```python
from build123d import *

# Parameters (mm, degrees)
BOSS_EXTRU_2_START = 2.33
ESQUISSE3_R        = 1
BOSS_EXTRU_2_DEPTH = 2.33
ESQUISSE4_R        = 0.9
BOSS_EXTRU_3_DEPTH = 2
ESQUISSE5_W        = 0.6
ESQUISSE5_H        = 4
PER_AGE1_D         = 1.47
PER_AGE1_DEPTH     = 1.6
CHANFREIN1_SIZE    = 0.1
CONG_1_R           = 0.2


# Read off the part's stored shape, not the designer's step: Boss.-Extru.1
with BuildPart() as part:
    # Esquisse1 → Révolution1 (revolve)
    with BuildSketch(Plane(origin=(0, 0, 0), x_dir=(1, 0, 0), z_dir=(0, 1, 0))):
        Polygon((1.175, 0.5), (0, 0.5), (0, -4.02), (0.799038106, -4.02), (1, -3.27), (1, -1.054421399), (1.02, -0.979780383), (1.02, -0.946167323), (1, -0.946167323), (1, 0), (1.175, 0), align=None)
    revolve(axis=Axis((0, 0, -0.5), (0, 0, 1)))

    # Boss.-Extru.1 outline → Boss.-Extru.1 (revolve)
    with BuildSketch(Plane.XZ):
        with BuildLine():
            Line((0.6, 4.02), (0.6, 6.37))
            ThreePointArc((0.6, 6.37), (0.424264069, 6.794264069), (0, 6.97))
            Line((0, 6.97), (0, 4.02))
            Line((0, 4.02), (0.6, 4.02))
        make_face()
    revolve(axis=Axis((0, 0, 0), (0, 0, 1)))

    # Esquisse3 → Boss.-Extru.2 (add)
    with BuildSketch(Plane(origin=(0, 0, -0.5), x_dir=(-1, 0, 0), z_dir=(0, 0, -1)).offset(BOSS_EXTRU_2_START)):
        with Locations(Location((0, 0, 0), (0, 0, 180))):
            Circle(ESQUISSE3_R)
    extrude(amount=-BOSS_EXTRU_2_DEPTH)

    # Esquisse4 → Boss.-Extru.3 (add)
    with BuildSketch(Plane(origin=(0, 0, -2.83), x_dir=(-1, 0, 0), z_dir=(0, 0, -1))):
        Circle(ESQUISSE4_R)
    extrude(amount=BOSS_EXTRU_3_DEPTH)

    # Esquisse5 → Enlèvement de matière-Révolution1 (revolve, cut)
    with BuildSketch(Plane(origin=(0, 0, 0), x_dir=(1, 0, 0), z_dir=(0, 1, 0)), mode=Mode.PRIVATE) as enl_vement_de_mati_re_r_volution1_sk:
        with Locations((0.3, -1.02)):
            Rectangle(ESQUISSE5_W, ESQUISSE5_H)
    revolve(enl_vement_de_mati_re_r_volution1_sk.sketch.rotate(Axis((0, 0, -0.98), (0, 0, 1)), 90), axis=Axis((0, 0, -0.98), (0, 0, 1)), mode=Mode.SUBTRACT)

    # Perçage1
    with Locations(Plane(origin=(0, 0, -4.83), x_dir=(-1, 0, 0), z_dir=(0, 0, -1))):
        with Locations((0, 0)):
            Hole(PER_AGE1_D / 2, depth=PER_AGE1_DEPTH)

    # Chanfrein1
    chanfrein1_edges = [part.edges().sort_by_distance(p)[0] for p in [
        (-0.735, 0, -4.83),
    ]]
    chamfer(chanfrein1_edges, length=CHANFREIN1_SIZE)

    # Congé1
    cong_1_edges = [part.edges().sort_by_distance(p)[0] for p in [
        (-0.799038106, 0, 4.02),
    ]]
    fillet(cong_1_edges, radius=CONG_1_R)


solid = part.part
```
Check sheet for the modelled part. Datum: model origin and axes. Units: mm. A direction names the side the tool comes from. Round coordinates to 2 decimals unless told otherwise and drop trailing zeros. Loops run counter-clockwise (first coordinate to the right, second up) from the corner with the lowest first, then second, coordinate; pieces in that order, holes last. Notation, with made-up numbers: (-8.75, -16) - (49.25, -16) arc R14 ccw to (49.25, -4) - close; hole circle Ø11 at (49, -39). An arc over 180 degrees is marked (long way). Answer as a JSON object with one key per item and string values. Group by question number.
Q1. Scan lines: line 1 along Y through (x, z) = (0, -4.3) (3 decimals); line 2 along Z through (x, y) = (-0.25, -0.6); line 3 along Z through (x, y) = (0, -0.45). Record each from-to range of solid material in increasing order. Write a range as [from, to].
Q2. Gauge pin test, flat ends, axial feed: P1, Ø0.6, axis at x = 0, y = 0, coming from the -Z side; P2, Ø1, axis at x = 0.5, z = 5, coming from the +Y side. Record the tip position at first contact, or that the pin passes through.
Q3. Mould release check, pull along Z, two halves, no side actions. Record for faces 5 (the face through (0, 0, 3.02)), 6 (the face through (0, 0, -3.23)), 7 (the face through (0, -1, 2)): released by +Z, released by -Z, zero draft, split by the parting line, or undercut.
Q4. Sectioned sample at A-A, the plane z = -3. Enter the section's corners in (x, y), plus the area to 3 significant figures.
Q5. Set-up check for faces 1 (the face through (0, 1, -2)), 2 (the face through (0.323, 0.506, 5.211)), 3 (the face through (-0.25, -1.15, -0.25)), 4 (the face through (-0.217, -0.976, 0.466)): record each of +Z, -Z, +X, -X, +Y, -Y from which the full face is reachable in a straight line by a thin tool's end or side.
Solution:
{
 "1": {"line 1": "y = [-0.9, -0.735], [0.735, 0.9]", "line 2": "z = [-3.23, 4.02]", "line 3": "z = [-3.23, -0.98], [3.02, 6.77]"},
 "2": {"P1": "stops at z = -3.23", "P2": "stops at y = 0.6"},
 "3": {"face 5": "undercut", "face 6": "released by -Z", "face 7": "zero draft"},
 "4": {"outline": "circle Ø1.8 at (0, 0)", "area": "2.54 mm²"},
 "5": {"face 1": "-Z", "face 2": "+Z", "face 3": "+Z, -Z", "face 4": "none"}
}
